The listing builds one solid part. Answer for the finished solid, in the listing's coordinates (mm). Face numbers are marked on the shaded views. A direction names the side the tool comes from. Round coordinates to 2 decimals unless told otherwise and drop trailing zeros. Loops run counter-clockwise (first coordinate to the right, second up) from the corner with the lowest first, then second, coordinate; pieces in that order, holes last. Notation, with made-up numbers: (36.25, -29) - (53.25, -29) arc R18 ccw to (53.25, -9) - close; hole circle Ø7 at (-35.5, -30.5). An arc over 180 degrees is marked (long way). Write item = value, one per line. Start each with the question number.
1) A tool of negligible diameter and unlimited length cuts with its end or side. For the marked faces 1, 2 and 3, from which of +Z, -Z, +X, -X, +Y, -Y can it reach the whole face along a straight path? Write none if from no direction.
2) Given pin 1 Ø3 at (x, y) = (40.5, 5.5) entering from +Z, flat-ended and moving along its own axis, determine where the tip first touches the part or whether it passes through.
3) Section C-C, the plane z = 4.5 is taken. Determine the outline of the cut face in (x, y).
4) Straight lines are drawn through the part: line 1 along Z through (x, y) = (28, 3); line 2 along X through (y, z) = (1.5, 1). For each, find the intervals that lie inside material, in ascending order.
5) Section A-A, the plane y = 1 is taken. Determine the outline of the cut face in (x, z).
6) Section B-B, the plane x = 28 is taken. Determine the outline of the cut face in (y, z), and give its area (3 significant figures).
from build123d import *

# Parameters (mm, degrees)
SKETCH1_W           = 12.7
SKETCH1_H           = 6.35
SKETCH1_W_2         = 50.8
SKETCH1_H_2         = 25.4
BOSS_EXTRUDE1_DEPTH = 6.35


with BuildPart() as part:
    # Sketch1 → Boss-Extrude1 (new body)
    with BuildSketch(Plane(origin=(0, 0, 0), x_dir=(1, 0, 0), z_dir=(0, 1, 0))):
        with Locations((19.05, -3.175)):
            Rectangle(SKETCH1_W, SKETCH1_H)
        with Locations((25.4, 12.7)):
            Rectangle(SKETCH1_W_2, SKETCH1_H_2)
    extrude(amount=BOSS_EXTRUDE1_DEPTH)


solid = part.part
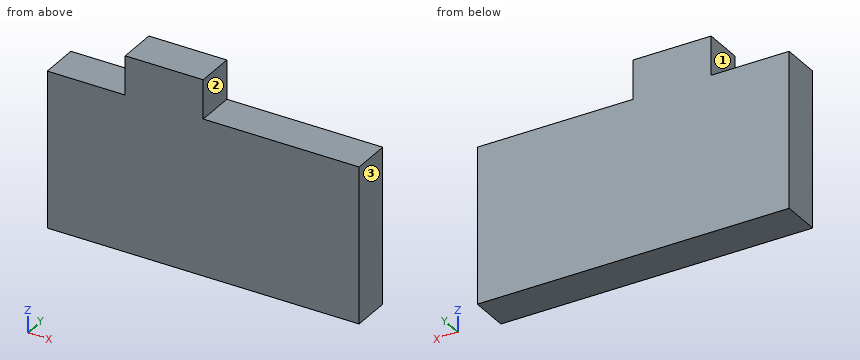
Geometry check:
q1.face_1 = +Z, -X, +Y, -Y
q1.face_2 = +Z, +X, +Y, -Y
q1.face_3 = +Z, -Z, +X, +Y, -Y
q2.pin_1 = 0
q3.outline = (12.7, 0) - (25.4, 0) - (25.4, 6.35) - (12.7, 6.35) - close
q4.line_1 = -25.4 to 0
q4.line_2 = 12.7 to 25.4
q5.outline = (0, -25.4) - (50.8, -25.4) - (50.8, 0) - (25.4, 0) - (25.4, 6.35) - (12.7, 6.35) - (12.7, 0) - (0, 0) - close
q6.outline = (0, -25.4) - (6.35, -25.4) - (6.35, 0) - (0, 0) - close
q6.area = 161 mm2
